Geometry check sheet. Reference: the model listing, model coordinates, mm. A direction names the side the tool comes from. Round coordinates to 2 decimals unless told otherwise and drop trailing zeros.
```python
from build123d import *

# Parameters (mm, degrees)
BOSS_EXTRUDE1_DEPTH = 3
SKETCH3_R           = 1.5
CUT_EXTRUDE2_DEPTH  = 3
CUT_EXTRUDE3_DEPTH  = 3


with BuildPart() as part:
    # Sketch1 → Boss-Extrude1 (new body)
    with BuildSketch(Plane(origin=(0, 0, 0), x_dir=(1, 0, 0), z_dir=(0, 1, 0))):
        Polygon((-5, 48), (5, 48), (5, 45), (15, 45), (15, 48), (25, 48), (25, 45), (35, 45), (35, 48), (45, 48), (45, 45), (55, 45), (55, 48), (65, 48), (65, 45), (75, 45), (75, 35), (78, 35), (78, 25), (75, 25), (75, 15), (78, 15), (78, 5), (75, 5), (75, -5), (78, -5), (78, -15), (75, -15), (75, -25), (78, -25), (78, -35), (75, -35), (75, -45), (65, -45), (65, -48), (55, -48), (55, -45), (45, -45), (45, -48), (35, -48), (35, -45), (25, -45), (25, -48), (15, -48), (15, -45), (5, -45), (5, -48), (-5, -48), (-5, -45), (-15, -45), (-15, -48), (-25, -48), (-25, -45), (-35, -45), (-35, -48), (-45, -48), (-45, -45), (-55, -45), (-55, -48), (-65, -48), (-65, -45), (-75, -45), (-75, -35), (-78, -35), (-78, -25), (-75, -25), (-75, -15), (-78, -15), (-78, -5), (-75, -5), (-75, 5), (-78, 5), (-78, 15), (-75, 15), (-75, 25), (-78, 25), (-78, 35), (-75, 35), (-75, 45), (-65, 45), (-65, 48), (-55, 48), (-55, 45), (-45, 45), (-45, 48), (-35, 48), (-35, 45), (-25, 45), (-25, 48), (-15, 48), (-15, 45), (-5, 45), align=None)
    extrude(amount=BOSS_EXTRUDE1_DEPTH)

    # Sketch3 → Cut-Extrude2 (cut)
    with BuildSketch(Plane(origin=(0, 3, 0), x_dir=(1, 0, 0), z_dir=(0, 1, 0))):
        with Locations(Location((41.5, -11.5, 0), (0, 0, 270))):
            Circle(SKETCH3_R)
        with Locations(Location((65, -11.5, 0), (0, 0, 270))):
            Circle(SKETCH3_R)
        with Locations(Location((65, -35, 0), (0, 0, 270))):
            Circle(SKETCH3_R)
        with Locations(Location((41.5, -35, 0), (0, 0, 270))):
            Circle(SKETCH3_R)
    extrude(amount=-CUT_EXTRUDE2_DEPTH, mode=Mode.SUBTRACT)

    # Sketch4 → Cut-Extrude3 (cut)
    with BuildSketch(Plane(origin=(0, 3, 0), x_dir=(1, 0, 0), z_dir=(0, 1, 0))):
        with BuildLine():
            Line((45, -35), (45, -38.5))
            Line((45, -38.5), (61.5, -38.5))
            Line((61.5, -38.5), (61.5, -35))
            ThreePointArc((61.5, -35), (62.525126266, -32.525126266), (65, -31.5))
            Line((65, -31.5), (68.5, -31.5))
            Line((68.5, -31.5), (68.5, -15))
            Line((68.5, -15), (65, -15))
            ThreePointArc((65, -15), (62.525126266, -13.974873734), (61.5, -11.5))
            Line((61.5, -11.5), (61.5, -8))
            Line((61.5, -8), (45, -8))
            Line((45, -8), (45, -11.5))
            ThreePointArc((45, -11.5), (43.974873734, -13.974873734), (41.5, -15))
            Line((41.5, -15), (38, -15))
            Line((38, -15), (38, -31.5))
            Line((38, -31.5), (41.5, -31.5))
            ThreePointArc((41.5, -31.5), (43.974873734, -32.525126266), (45, -35))
        make_face()
    extrude(amount=-CUT_EXTRUDE3_DEPTH, mode=Mode.SUBTRACT)


solid = part.part
```
(1) Material ranges on line 1 (X direction, y = 2.35, z = 11.5); line 2 (X direction, y = 0.7, z = 26); line 3 (X direction, y = 1.1, z = 22), recorded low to high.
Returned:
line 1: x = -78 to 40, 43 to 45, 61.5 to 63.5, 66.5 to 78
line 2: x = -78 to 38, 68.5 to 78
line 3: x = -75 to 38, 68.5 to 75
(2) Depth check by flat-ended pin: P1, Ø1.5, axis at x = 11.5, y = 2, coming from the -Z side; P2, Ø1.5, axis at y = 1, z = 39, coming from the +X side; P3, Ø1.5, axis at y = 2, z = 46.5, coming from the -X side. Enter the tip coordinate at first touch or a pass-through.
Returned:
P1: stops at z = -45
P2: stops at x = 75
P3: stops at x = -65
(3) Set-up check for faces 1 (the flat face through (77, 1, 15)), 2 (the flat face through (-45, 1, -46)), 3 (the flat face through (-65, 1, -46)), 4 (the flat face through (76, 1, -35)), 5 (the flat face through (67, 2, 31.5)): record each of +Z, -Z, +X, -X, +Y, -Y from which the full face is reachable in a straight line by a thin tool's end or side.
Returned:
face 1: +X, +Y, -Y
face 2: -Z, +Y, -Y
face 3: -Z, -X, +Y, -Y
face 4: -Z, +X, +Y, -Y
face 5: +Y, -Y
(4) Sectioned sample at A-A, the plane y = 2.4. Give the number of separate pieces and of enclosed holes in the cut face, and give its area (3 significant figures).
Returned:
separate pieces: 1
enclosed holes: 5
area: 13,400 mm2
(5) Draft check along Z on faces 6 (the flat face through (-40, 1, -48)), 7 (the flat face through (-75, 1, 20)), 8 (the flat face through (-65, 1, 47)), 9 (the cylindrical face through (62.5, 1.52, 32.55)). Enter one of: released by +Z, released by -Z, zero draft, split by the parting line, or undercut.
Returned:
face 6: released by -Z
face 7: undercut
face 8: zero draft
face 9: undercut
